Can you work these out from the model? Positions are in its coordinate system, mm. Face numbers are marked on the shaded views. Round coordinates to 2 decimals unless told otherwise and drop trailing zeros. Order: outer loops, then holes, each group sorted by start corner. A loop starts at its lowest first (then second) coordinate and runs counter-clockwise, first axis right, second up.
Q1. If we section it at A-A (x = 5.75): Please give me the cut outline in (y, z).
Q2. We'd pull the mould along Y, two halves only. Please class the marked faces 1, 2, 3 and 4: pulls with the +Y half, pulls with the -Y half, needs draft (parallel to the pull), parting line crosses it, or undercut.
Q3. Will these pins go through, and if not, where does the flat tip stop? P1, Ø2, axis at x = 7, z = 1, coming from the +Y side; P2, Ø2, axis at x = 3, y = 2, coming from the +Z side; P3, Ø3, axis at x = 5, z = 2.5, coming from the -Y side.
Q4. If I drill on line 1 (Z direction, x = 9, y = 1.25); line 2 (Y direction, x = 7.75, z = -0.25); line 3 (Z direction, x = 11.5, y = -0.5), over which ranges is the centre line in solid material (lowest first)?
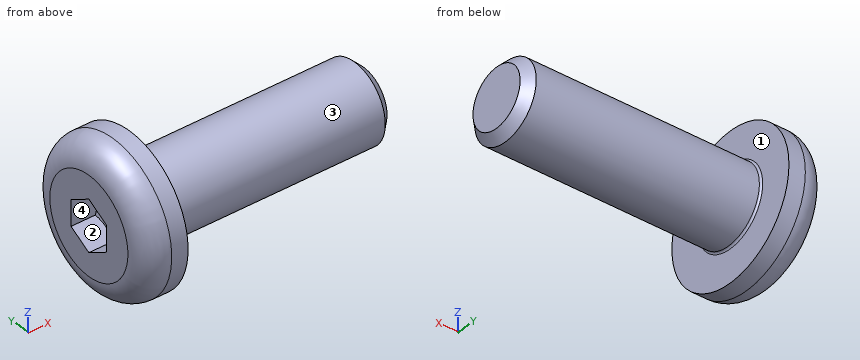
Autodesk Inventor part; units mm, degrees
ref_plane "Work Plane1" through (29, 0, 0) normal (0, -1, 0) x (1, 0, 0)
ref_plane "YZ Plane" through (0, 0, 0) normal (1, 0, 0) x (0, 1, 0)
ref_plane "XZ Plane" through (0, 0, 0) normal (0, 1, 0) x (-1, 0, 0)
sketch "Sketch1" plane through (0, 0, 0) normal (0, 0, 1) x (1, 0, 0)
  line L0 (-0.0847, 0) -> (12.7, 0)
  line L1 (12.7, 0) -> (12.7, 2.0828)
  line L2 (12.7, 2.0828) -> (1.5242, 2.0828)
  line L3 (1.5242, 2.0828) -> (0.0001, 2.0828)
  line L4 (0.0001, 2.0828) -> (0, 2.0828)
  line L5 (0, 2.0828) -> (0, 3.9624)
  line L6 (0, 3.9624) -> (-2.2098, 3.9624)
  line L7 (-2.2098, 3.9624) -> (-2.2098, 1.3931)
  line L8 (-2.2098, 1.3931) -> (-0.889, 1.3931)
  line L9 (-0.889, 1.3931) -> (-0.0847, 0)
  line L10 (-5.1918, 0) -> (15.682, 0)
  line L11 (0, -0.7925) -> (0, 4.7549)
  line L12 (1.5242, 2.0828) -> (0, 2.0828) construction
  dimension "d1" = 11.1758
  dimension "d2" = 1.5241
  dimension "d3" = 2.2098
  dimension "d4" = 1.3208
  dimension "d5" = 60
  dimension "d6" = 4.1656
  dimension "d7" = 4.1656
  dimension "d8" = 2.7863
  dimension "d9" = 7.9248
  dimension "d26" = 12.7
revolve "Body" add sketch "Sketch1" angle 360 about axis through (-0.0847, 0, 0) along (1, 0, 0)
sketch "Sketch2" plane through (-2.2098, 0, 0) normal (-1, 0, 0) x (0, 0, 1)
  circle A0 centre (0, 0) radius 1.3931
  line L0 (0, -5.5474) -> (0, 5.5474)
  line L1 (-5.5474, 0) -> (5.5474, 0)
  line L2 (1.3931, 0) -> (0.6966, -1.2065)
  line L3 (0.6966, -1.2065) -> (-0.6966, -1.2065)
  line L4 (-0.6966, -1.2065) -> (-1.3931, 0)
  line L5 (-1.3931, 0) -> (-0.6966, 1.2065)
  line L6 (-0.6966, 1.2065) -> (0.6966, 1.2065)
  line L7 (0.6966, 1.2065) -> (1.3931, 0)
extrude "Slot" add sketch "Sketch2" against normal up to next contours L7 A0 | A0 L2 | L6 L0 A0 | A0 L0 L3 | L0 L6 A0 | A0 L3 L0 | L4 A0 | A0 L5
fillet "Fillet1" radius 1.3208 1 edges at (-2.2098, -3.9624, 0)
thread "Thread"
chamfer "Chamfer1" distance 0.4869 distance2 0.4869 1 edges at (12.7, -2.0828, 0) measured on face at (12.7, -0.1898, 0.4203)
ref_plane "Work Plane1" through (29, 0, 0) normal (0, -1, 0) x (1, 0, 0)
fillet "Fillet2" radius 0.1 1 edges at (0.0001, -2.0828, 0)
equation "\"d30\" = R"
equation "\"d17\" = RR"
equation "\"d13\" = GEL"
equation "\"d15\" = -0.5 * SPD + 0.5 * GD"
equation "\"d16\" = GUL"
equation "\"d1\" = GEL"
equation "\"d3\" = KOH"
equation "\"d4\" = INTI"
equation "\"d6\" = GD"
equation "\"d7\" = BDM"
equation "\"d8\" = 1.1547 * SW"
equation "\"d9\" = KOD"
equation "\"d26\" = NLG"
equation "\"GD\" = NND"
equation "\"NLG\" = 12.7"
equation "\"GEL\" = 11.1758"
equation "\"KOD\" = 7.9248"
equation "\"KOH\" = 2.2098"
equation "\"INTI\" = 1.3208"
equation "\"GAL\" = 1.524"
equation "\"GUL\" = 0.48692"
equation "\"BDM\" = NND"
equation "\"SW\" = 2.413"
equation "\"RR\" = 1.3208"
equation "\"SPD\" = GD1"
equation "\"R\" = 0.1"
equation "\"KR\" = 4.699"
equation "\"GD1\" = 3.19177"
equation "\"THREADDIA\" = 4.1656"
equation "\"FAWI\" = 45deg"
equation "\"KOH1\" = 1.3208"
equation "\"NND\" = 4.1656"
equation "\"TOA\" = 30deg"
equation "\"E0\" = 1.155 * SW"
properties part number "Unbrako - 8 x 1/2" material "Steel, Mild"
Solution:
1. outline: circle Ø4.17 at (0, 0)
2. face 1: needs draft
2. face 2: undercut
2. face 3: parting line crosses it
2. face 4: undercut
3. P1: stops at y = 2.08
3. P2: stops at z = 1.83
3. P3: stops at y = -1.83
4. line 1: z = -1.67 to 1.67
4. line 2: y = -2.07 to 2.07
4. line 3: z = -2.02 to 2.02
